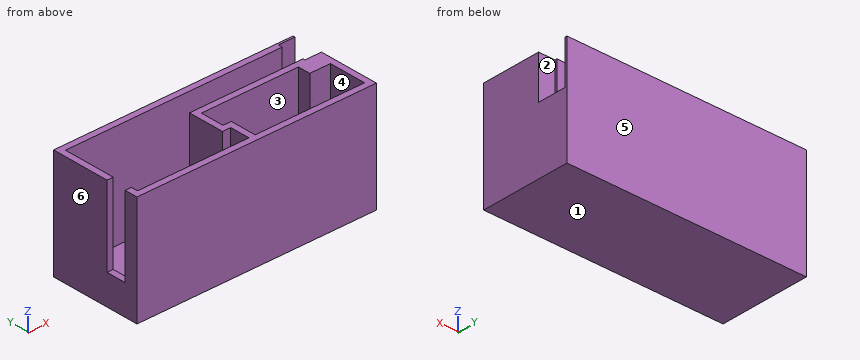
from build123d import *

# Parameters (mm, degrees)
SKETCH1_W           = 58
SKETCH1_H           = 22
BOSS_EXTRUDE1_DEPTH = 1.5
SKETCH2_W           = 58
SKETCH2_H           = 22
BOSS_EXTRUDE2_DEPTH = 25
CUT_EXTRUDE1_DEPTH  = 5
SKETCH6_W           = 10.5
SKETCH6_H           = 7
CUT_EXTRUDE2_DEPTH  = 4


with BuildPart() as part:
    # Sketch1 → Boss-Extrude1 (new body)
    with BuildSketch(Plane.XY):
        with Locations((9.718487395, 11)):
            Rectangle(SKETCH1_W, SKETCH1_H)
    extrude(amount=BOSS_EXTRUDE1_DEPTH)

    # Sketch2 → Boss-Extrude2 (add)
    with BuildSketch(Plane.XY.offset(1.5)):
        with Locations((9.718487395, 11)):
            Rectangle(SKETCH2_W, SKETCH2_H)
        Polygon((-17.781512605, 20.5), (-17.781512605, 1.5), (9.218487395, 1.5), (9.218487395, 6.3), (7.218487395, 6.3), (7.218487395, 15), (37.218487395, 15), (37.218487395, 20.5), align=None, mode=Mode.SUBTRACT)
        Polygon((37.218487395, 1.5), (37.218487395, 10.5), (32.218487395, 10.5), (32.218487395, 13.5), (8.718487395, 13.5), (8.718487395, 7.8), (10.718487395, 7.8), (10.718487395, 1.5), align=None, mode=Mode.SUBTRACT)
    extrude(amount=BOSS_EXTRUDE2_DEPTH)

    # Sketch3 → Cut-Extrude1 (cut)
    with BuildSketch(Plane.ZY.offset(19.281512605)):
        Polygon((7.25, 3.1), (19.25, 3.1), (26.5, 3.1), (26.5, 7.9), (19.25, 7.9), (7.25, 7.9), align=None)
    extrude(amount=-CUT_EXTRUDE1_DEPTH, mode=Mode.SUBTRACT)

    # Sketch6 → Cut-Extrude2 (cut)
    with BuildSketch(Plane(origin=(38.718487395, 0, 0), x_dir=(0, 0, -1), z_dir=(1, 0, 0))):
        with Locations((-21.25, 18)):
            Rectangle(SKETCH6_W, SKETCH6_H)
    extrude(amount=-CUT_EXTRUDE2_DEPTH, mode=Mode.SUBTRACT)


solid = part.part
Part model, mm, in its own coordinate system. Face numbers are marked on the shaded views. A direction names the side the tool comes from. Round coordinates to 2 decimals unless told otherwise and drop trailing zeros. Write each loop counter-clockwise with the first axis right and the second up, starting at its lowest first coordinate (ties: lowest second). Pieces come first, ordered by that corner, then holes. Notation, with made-up numbers: (-12, 35.25) - (42, 35.25) arc R5 ccw to (42, 42.25) - close; hole circle Ø3 at (-15, 56). An arc over 180 degrees is marked (long way). Use CSV: the item, a comma, the result in double quotes.
Item 1: Slice it at A-A, the plane z = 17. Write the cut outline in (x, y), then the cut area to 3 significant figures.
Results list:
outline,"(-19.28, 0) - (38.72, 0) - (38.72, 14.5) - (34.72, 14.5) - (34.72, 15) - (7.22, 15) - (7.22, 6.3) - (9.22, 6.3) - (9.22, 1.5) - (-17.78, 1.5) - (-17.78, 3.1) - (-19.28, 3.1) - close; (-19.28, 7.9) - (-17.78, 7.9) - (-17.78, 20.5) - (34.72, 20.5) - (34.72, 21.5) - (38.72, 21.5) - (38.72, 22) - (-19.28, 22) - close; hole (8.72, 7.8) - (10.72, 7.8) - (10.72, 1.5) - (37.22, 1.5) - (37.22, 10.5) - (32.22, 10.5) - (32.22, 13.5) - (8.72, 13.5) - close"
area,"291 mm²"
Item 2: Slice it at B-B, the plane z = 2.25. Write the cut outline in (x, y).
Results list:
outline,"(-19.28, 0) - (38.72, 0) - (38.72, 22) - (-19.28, 22) - close; hole (-17.78, 1.5) - (9.22, 1.5) - (9.22, 6.3) - (7.22, 6.3) - (7.22, 15) - (37.22, 15) - (37.22, 20.5) - (-17.78, 20.5) - close; hole (8.72, 7.8) - (10.72, 7.8) - (10.72, 1.5) - (37.22, 1.5) - (37.22, 10.5) - (32.22, 10.5) - (32.22, 13.5) - (8.72, 13.5) - close"
Item 3: Wall check: L1, parallel to Y at x = 22, z = 17; L2, parallel to Y at x = 9.5, z = 22.75; L3, parallel to X at y = 11.25, z = 25. Give the ranges that are in metal, low to high.
Results list:
L1,"y = 0 to 1.5, 13.5 to 15, 20.5 to 22"
L2,"y = 0 to 7.8, 13.5 to 15, 20.5 to 22"
L3,"x = -19.28 to -17.78, 7.22 to 8.72, 32.22 to 38.72"
Item 4: Slice it at C-C, the plane y = 11.25. Write the cut outline in (x, z), then the cut area to 4 significant figures.
Results list:
outline,"(-19.28, 0) - (38.72, 0) - (38.72, 26.5) - (32.22, 26.5) - (32.22, 1.5) - (8.72, 1.5) - (8.72, 26.5) - (7.22, 26.5) - (7.22, 1.5) - (-17.78, 1.5) - (-17.78, 26.5) - (-19.28, 26.5) - close"
area,"324.5 mm²"
Item 5: Flat gauge pins, fed straight in: P1, Ø2.5, axis at y = 5, z = 19.5, coming from the -X side; P2, Ø3, axis at x = 36, y = 17.5, coming from the +Z side. Where does each tip first touch, or does it go through?
Results list:
P1,"stops at x = 9.22"
P2,"stops at z = 16"
Item 6: Tool access for the marked faces 1, 2 and 3: list every direction of +Z, -Z, +X, -X, +Y, -Y with a clear straight run to the whole face (end or side of a thin tool).
Results list:
face 1,"-Z, +X, -X, +Y, -Y"
face 2,"+Z, +X"
face 3,"+Z"
Item 7: Pull direction X, two halves, no side cores. Call the marked faces 4, 5 and 6: pulls with the +X half, pulls with the -X half, needs draft (parallel to the pull), parting line crosses it, or undercut.
Results list:
face 4,"undercut"
face 5,"needs draft"
face 6,"pulls with the -X half"
Item 8: Slice it at D-D, the plane x = 26.5. Write the cut outline in (y, z).
Results list:
outline,"(0, 0) - (22, 0) - (22, 26.5) - (20.5, 26.5) - (20.5, 1.5) - (15, 1.5) - (15, 26.5) - (13.5, 26.5) - (13.5, 1.5) - (1.5, 1.5) - (1.5, 26.5) - (0, 26.5) - close"
